For this review, take the finished solid that the model builds, in its own axes (mm). A direction names the side the tool comes from. Coordinates: 2 decimals unless noted, no trailing zeros. Write each loop counter-clockwise with the first axis right and the second up, starting at its lowest first coordinate (ties: lowest second). Pieces come first, ordered by that corner, then holes. Notation, with made-up numbers: M 75.25,49.25 L 127.25,49.25 A27 ccw 127.25,80.25 Z; hole C 51.5,63 d1. An arc over 180 degrees is marked long. Return JSON: item names as keys, results as strings.
Autodesk Inventor part; units mm, degrees
ref_plane "YZ Plane" through (0, 0, 0) normal (1, 0, 0) x (0, 1, 0)
ref_plane "XZ Plane" through (0, 0, 0) normal (0, 1, 0) x (-1, 0, 0)
ref_plane "XY Plane" through (0, 0, 0) normal (0, 0, 1) x (1, 0, 0)
sketch "Эскиз1" plane through (0, 0, 0) normal (0, 1, 0) x (-1, 0, 0)
  line L0 (0, 0) -> (3, 0)
  line L1 (3, 0) -> (3, -3)
  line L2 (3, -3) -> (0, -3)
  line L3 (0, -3) -> (0, 0)
  line L4 (3, 0) -> (20, 0)
  line L5 (20, 0) -> (17, 0)
  line L6 (17, 0) -> (17, -3)
  line L7 (17, -3) -> (20, -3)
  line L8 (20, -3) -> (20, 0)
  line L9 (20, 0) -> (37, 0)
  line L10 (37, 0) -> (34, 0)
  line L11 (34, 0) -> (34, -3)
  line L12 (34, -3) -> (37, -3)
  line L13 (37, -3) -> (37, 0)
  line L14 (37, 0) -> (54, 0)
  line L15 (54, 0) -> (51, 0)
  line L16 (51, 0) -> (51, -3)
  line L17 (51, -3) -> (54, -3)
  line L18 (54, -3) -> (54, 0)
  point P0 (17, 0)
  point P1 (17, 0)
  dimension "d0" = 3
  dimension "d1" = 3
  dimension "d17" = 17
  dimension "d18" = 3
  dimension "d19" = 3
  dimension "d20" = 17
  dimension "d21" = 17
  dimension "d22" = 3
  dimension "d23" = 3
  dimension "d24" = 3
  dimension "d25" = 3
extrude "Выдавливание1" add sketch "Эскиз1" along normal blind 4
sketch "Эскиз2" plane through (0, 4, 0) normal (0, 1, 0) x (1, 0, 0)
  line L0 (0, 0) -> (-90, 0)
  line L1 (-90, 0) -> (-90, 3)
  line L2 (-90, 3) -> (0, 3)
  line L3 (0, 3) -> (0, 0)
  dimension "d13" = 3
  dimension "d14" = 90
extrude "Выдавливание2" add sketch "Эскиз2" along normal blind 15
fillet "Сопряжение1" radius 1 1 edges at (-17, 4, -1.5)
fillet "Сопряжение2" radius 2 7 edges at (-34, 4, -1.5) (-51, 4, -1.5) (-54, 4, -1.5) (-37, 4, -1.5) (-20, 4, -1.5) (-3, 4, -1.5) (0, 19, -1.5)
fillet "Сопряжение3" radius 2 2 edges at (-90, 19, -1.5) (-90, 4, -1.5)
properties part number "Bus_copper_GND" material "Медь"
1. Wall thickness on L1, parallel to X at y = 2, z = -1.3; L2, parallel to X at y = 3, z = -2.45; L3, parallel to Y at x = -43.5, z = -0.25: over which ranges is each line inside the solid? List them lowest first. Write a range as from..to.
Checks:
{"L1": "-54..-51, -37..-34, -20..-17, -3..0", "L2": "-54.27..-50.73, -37.27..-33.73, -20.27..-17, -3.27..0", "L3": "4..19"}
2. For faces 1 (the face through (-54, 1, -2)), 2 (the face through (-18, 0, -1)), 3 (the face through (-27, 4, -2)), list the 3-axis set-ups (+Z, -Z, +X, -X, +Y, -Y) from which the entire face can be reached by the end or side of a thin tool; tool diameter is ignored.
Checks:
{"face 1": "+Z, -Z, -X, -Y", "face 2": "+Z, -Z, +X, -X, -Y", "face 3": "+Z, -Z, -Y"}
3. Clearance check with flat-ended pins moving along their axes: pin 1 Ø1.5 at (x, z) = (-75.5, -1.5) entering from -Y; pin 2 Ø1.6 at (y, z) = (1.5, -1.5) entering from -X. State where each tip first meets the part, or that it passes through.
Checks:
{"pin 1": "y = 4", "pin 2": "x = -54.02"}
4. Draft analysis for pull direction X (two halves, no side actions). For faces 4 (the face through (-11, 4, -2)), 5 (the face through (-1, 0, -1)), 6 (the face through (-54.57, 3.4, -1.48)), 7 (the face through (-17, 1, -1)), state which applies: +X half, -X half, draft (parallel to the pull), parting line (faces both ways), or undercut.
Checks:
{"face 4": "undercut", "face 5": "draft", "face 6": "-X half", "face 7": "undercut"}
5. We need section B-B (x = -65). State the section outline as (y, z) points, plus the area to 3 significant figures.
Checks:
{"outline": "M 4,-3 L 19,-3 L 19,0 L 4,0 Z", "area": "45.0 mm2"}
6. We need section A-A (z = -0.7). State the section outline as (x, y) points.
Checks:
{"outline": "M -90,6 A2 ccw -88,4 L -56,4 A2 cw -54,2 L -54,0 L -51,0 L -51,2 A2 cw -49,4 L -39,4 A2 cw -37,2 L -37,0 L -34,0 L -34,2 A2 cw -32,4 L -22,4 A2 cw -20,2 L -20,0 L -17,0 L -17,3 A1 cw -16,4 L -5,4 A2 cw -3,2 L -3,0 L 0,0 L 0,17 A2 ccw -2,19 L -88,19 A2 ccw -90,17 Z"}
